For this review, take the finished solid that the model builds, in its own axes (mm). Round coordinates to 2 decimals unless told otherwise and drop trailing zeros. Write each loop counter-clockwise with the first axis right and the second up, starting at its lowest first coordinate (ties: lowest second). Pieces come first, ordered by that corner, then holes. Notation, with made-up numbers: M 20.5,7 L 58.5,7 A31 ccw 58.5,46 Z; hole C -28,5 d11. An arc over 180 degrees is marked long. Use one line per item in the form item = value. Start each with the question number.
Item 1: Draft analysis for pull direction Y (two halves, no side actions). For faces 1 (the flat face through (15, 1, 7)), 2 (the cylindrical face through (-39.383, 41.67, 3.451)), 3 (the cylindrical face through (69.15, -21.78, 3.45)), state which applies: released by +Y, released by -Y, zero draft, split by the parting line, or undercut.
Item 2: Add section D-D (y = 7.5). State the section outline as (x, z) points.
Item 3: Add section C-C (y = 25). State the section outline as (x, z) points, and give its area (3 significant figures).
Item 4: For P1, Ø3.5, axis at x = 0, y = -29, coming from the +Z side; P2, Ø3, axis at y = -30, z = 5.5, coming from the +X side; P3, Ø1, axis at x = -52.5, z = 5, coming from the -Y side, all flat-tipped, find the tip position at first contact; note any pin that passes through.
Item 5: Add section B-B (x = 0). State the section outline as (y, z) points, and give its area (3 significant figures).
Item 6: Add section A-A (z = 1.5). Count the separate pieces of the cut face and the enclosed holes in it, and give its area (3 significant figures).
Item 7: For line 1 (Y direction, x = 2.5, z = 4.5); line 2 (Y direction, x = 2, z = 1); line 3 (Y direction, x = -41, z = 4.5), list the stretches that pass through material, from the lowest coordinate up. Write a range as [from, to].
Autodesk Inventor part; units mm, degrees
ref_plane "YZ Plane" through (0, 0, 0) normal (1, 0, 0) x (0, 1, 0)
ref_plane "XZ Plane" through (0, 0, 0) normal (0, 1, 0) x (-1, 0, 0)
ref_plane "XY Plane" through (0, 0, 0) normal (0, 0, 1) x (1, 0, 0)
sketch "Sketch1" plane through (0, 0, 0) normal (0, 0, 1) x (1, 0, 0)
  circle A0 centre (0, 0) radius 72.5
  line L0 (-41, 0) -> (41, 0) construction
  line L1 (0, -41) -> (0, 41) construction
  line L2 (0, 41) -> (41, 41) construction
  line L3 (41, 41) -> (41, 0) construction
  circle A1 centre (41, 41) radius 1.75
  circle A2 centre (41, -41) radius 1.75
  circle A3 centre (-41, 41) radius 1.75
  circle A4 centre (-41, -41) radius 1.75
  circle A5 centre (41, 41) radius 5 construction
  circle A6 centre (41, -41) radius 5 construction
  circle A7 centre (-41, -41) radius 5 construction
  circle A8 centre (-41, 41) radius 5 construction
  line L4 (0, 0) -> (0, -45) construction
  circle A9 centre (0, 0) radius 45 construction
  circle A10 centre (0, 0) radius 11
  circle A11 centre (0, -45) radius 5.1
  line L5 (0, -61) -> (0, -29) construction
  circle A12 centre (0, -61) radius 2.25
  circle A13 centre (0, -29) radius 2.25
  circle A14 centre (52.8275, 30.5) radius 2.25
  line L6 (52.8275, 30.5) -> (25.1147, 14.5) construction
  circle A15 centre (38.9711, 22.5) radius 5.1
  circle A16 centre (25.1147, 14.5) radius 2.25
  circle A17 centre (-52.8275, 30.5) radius 2.25
  line L7 (-52.8275, 30.5) -> (-25.1147, 14.5) construction
  circle A18 centre (-38.9711, 22.5) radius 5.1
  circle A19 centre (-25.1147, 14.5) radius 2.25
  point P0 (38.9711, 22.5)
  dimension "d0" = 145
  dimension "L_furos" = 82
  dimension "d2" = 82
  dimension "d3" = 3.5
  dimension "d4" = 10
  dimension "d5" = 45
  dimension "d24" = 360
  dimension "d49" = 22
  dimension "d52" = 10.2
  dimension "d54" = 32
  dimension "d55" = 4.5
  dimension "d56" = 4.5
  dimension "d59" = 360
extrude "Extrusion1" add sketch "Sketch1" along normal blind 7
equation "\"d2\" = L_furos"
equation "\"d21\" = 5.5"
equation "\"d39\" = 5.5"
properties part number "SupBase"
Calculated:
q1.face_1 = zero draft
q1.face_2 = undercut
q1.face_3 = split by the parting line
q2.outline = M -72.11,0 L -8.05,0 L -8.05,7 L -72.11,7 Z; M 8.05,0 L 72.11,0 L 72.11,7 L 8.05,7 Z
q3.outline = M -68.05,0 L -43.42,0 L -43.42,7 L -68.05,7 Z; M -34.53,0 L 34.53,0 L 34.53,7 L -34.53,7 Z; M 43.42,0 L 68.05,0 L 68.05,7 L 43.42,7 Z
q3.area = 828 mm^2
q4.P1 = through
q4.P2 = 66.66
q4.P3 = -50.52
q5.outline = M -72.5,0 L -63.25,0 L -63.25,7 L -72.5,7 Z; M -58.75,0 L -50.1,0 L -50.1,7 L -58.75,7 Z; M -39.9,0 L -31.25,0 L -31.25,7 L -39.9,7 Z; M -26.75,0 L -11,0 L -11,7 L -26.75,7 Z; M 11,0 L 72.5,0 L 72.5,7 L 11,7 Z
q5.area = 727 mm^2
q6.separate_pieces = 1
q6.enclosed_holes = 14
q6.area = 15,800 mm^2
q7.line_1 = [-72.46, -49.45], [-40.55, -10.71], [10.71, 72.46]
q7.line_2 = [-72.47, -62.03], [-59.97, -49.69], [-40.31, -30.03], [-27.97, -10.82], [10.82, 72.47]
q7.line_3 = [-59.79, -42.75], [-39.25, 17.82], [27.18, 39.25], [42.75, 59.79]
